Geometry check sheet. Reference: drawing and pictorial views, mm from the part's lowest x, y, z. A direction names the side the tool comes from. Give positions to 0.01 mm unless a question says otherwise; leave off trailing zeros. Order: outer loops, then holes, each group sorted by start corner. A loop starts at its lowest first (then second) coordinate and runs counter-clockwise, first axis right, second up.
Item 1: Sectioned sample at A-A on x = 10.85. Record the boundary of the cut face in (y, z) (3 decimals).
Item 2: Material ranges on line 1 along X through (y, z) = (10.85, 11.5) (3 decimals); line 2 along Z through (x, y) = (8.5, 18), recorded low to high.
Item 3: Access from +Z, -Z, +X, -X, +Y, -Y to the whole of each face (thin tool, end or side, straight path). Record for the marked faces 1, 2 and 3.
Item 4: Sectioned sample at D-D on y = 2.5. Record the boundary of the cut face in (x, z), and give its area (3 significant figures).
Item 5: Gauge pin test, flat ends, axial feed: P1, Ø2, axis at y = 7, z = 15, coming from the +X side; P2, Ø8, axis at y = 15.5, z = 9, coming from the +X side; P3, Ø4, axis at x = 10, z = 14.5, coming from the +Y side (3 decimals); P4, Ø6, axis at x = 6, z = 2.5, coming from the +Y side. Record the tip position at first contact, or that the pin passes through.
Item 6: Sectioned sample at C-C on z = 3. Record the boundary of the cut face in (x, y).
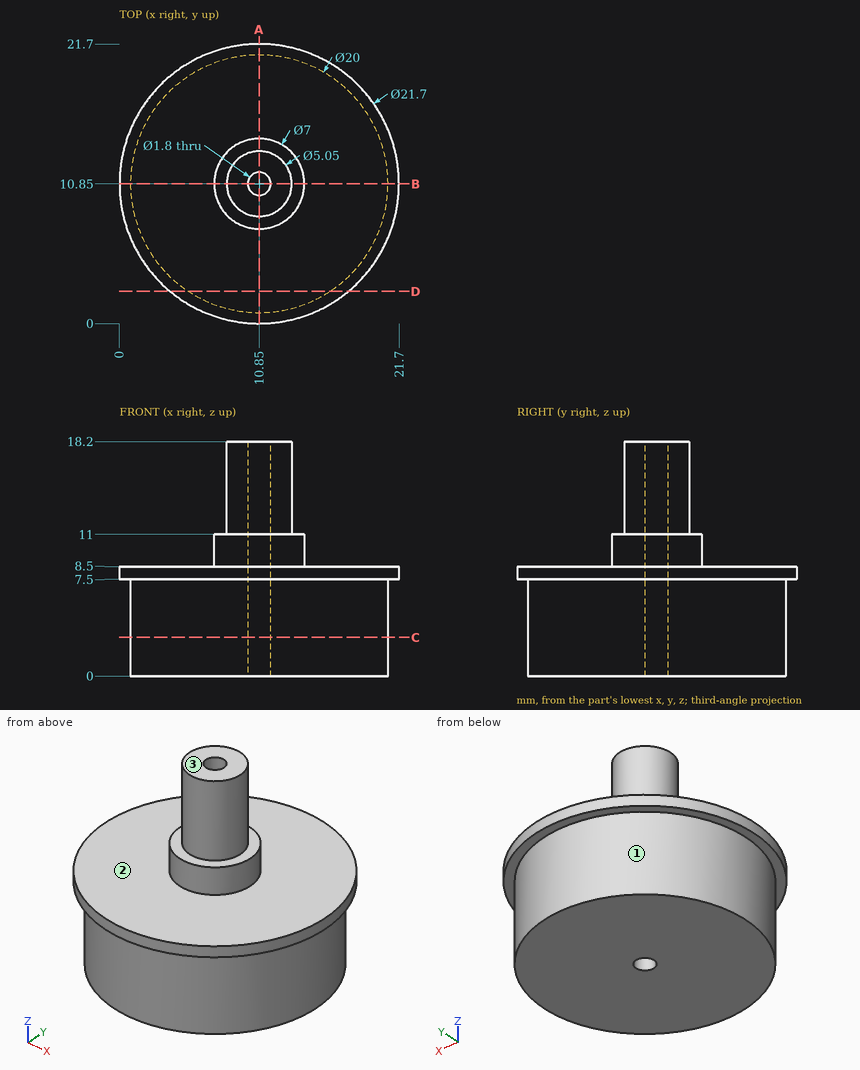
Report:
1. outline: (0, 7.5) - (0.85, 7.5) - (0.85, 0) - (9.95, 0) - (9.95, 18.2) - (8.325, 18.2) - (8.325, 11) - (7.35, 11) - (7.35, 8.5) - (0, 8.5) - close; (11.75, 0) - (20.85, 0) - (20.85, 7.5) - (21.7, 7.5) - (21.7, 8.5) - (14.35, 8.5) - (14.35, 11) - (13.375, 11) - (13.375, 18.2) - (11.75, 18.2) - close
2. line 1: x = 8.325 to 9.95, 11.75 to 13.375
2. line 2: z = 0 to 8.5
3. face 1: -Z
3. face 2: +Z
3. face 3: +Z, +X, -X, +Y, -Y
4. outline: (3.92, 7.5) - (5.35, 7.5) - (5.35, 0) - (16.35, 0) - (16.35, 7.5) - (17.78, 7.5) - (17.78, 8.5) - (3.92, 8.5) - close
4. area: 96.4 mm2
5. P1: passes through
5. P2: stops at x = 21.68
5. P3: stops at y = 13.375
5. P4: stops at y = 20.68
6. outline: circle Ø20 at (10.85, 10.85); hole circle Ø1.8 at (10.85, 10.85)
